Can you work these out from the model? Positions are in its coordinate system, mm. Round coordinates to 2 decimals unless told otherwise and drop trailing zeros. Loops run counter-clockwise (first coordinate to the right, second up) from the corner with the lowest first, then second, coordinate; pieces in that order, holes last. Notation, with made-up numbers: M -29.5,-12 L 2.5,-12 A8 cw 2.5,-5 Z; hole C 89,27 d9. An arc over 180 degrees is marked long. Answer as CSV lines item,"result".
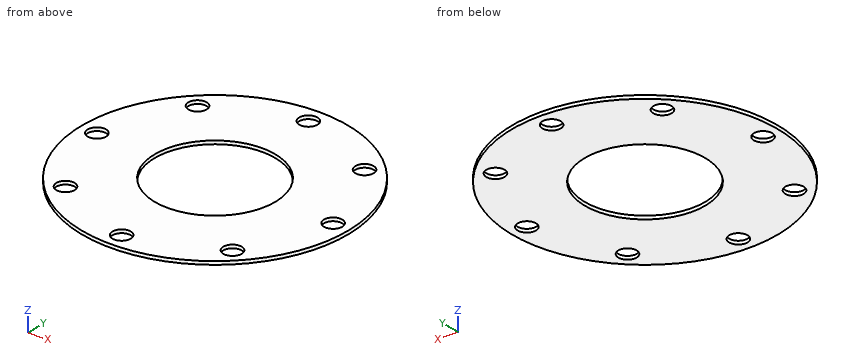
Autodesk Inventor part; units mm, degrees
ref_plane "YZ Plane" through (0, 0, 0) normal (1, 0, 0) x (0, 1, 0)
ref_plane "XZ Plane" through (0, 0, 0) normal (0, 1, 0) x (-1, 0, 0)
ref_plane "XY Plane" through (0, 0, 0) normal (0, 0, 1) x (1, 0, 0)
sketch "Sketch1" plane through (0, 0, 0) normal (0, 0, 1) x (1, 0, 0)
  circle A0 centre (0, 0) radius 72.5
  circle A1 centre (0, 0) radius 160
  dimension "d22" = 145
  dimension "d23" = 320
extrude "Plate1" add sketch "Sketch1" along normal blind 4
sketch "Sketch5" plane through (0, 0, 4) normal (0, 0, 1) x (1, 0, 0)
  circle A0 centre (0, 140) radius 11
  circle A1 centre (0, 0) radius 140 construction
  circle A2 centre (0, 0) radius 190 construction
  circle A3 centre (0, 190) radius 6.5
  dimension "d25" = 280
  dimension "d32" = 380
  dimension "d24" = 22
  dimension "d31" = 13
extrude "Cut1" cut sketch "Sketch5" against normal blind 4 contours A0
pattern_circular "Circular Pattern1" count 8 over 360 about axis through (0, 0, 0) along (0, 0, 1) of "Cut1"
equation "\"d26\" = Thickness"
equation "\"d2\" = Thickness"
equation "\"BendReliefWidth\" = Thickness"
equation "\"BendReliefDepth\" = 0.5 * Thickness"
equation "\"CornerReliefSize\" = 4 * Thickness"
equation "\"MinimumRemnant\" = 2 * Thickness"
equation "\"TransitionRadius\" = BendRadius"
equation "\"JacobiRadiusSize\" = BendRadius"
equation "\"GapSize\" = Thickness"
properties part number "TKS 3109 top DS main flange" material "Stainless Steel"
Item 1: If we section it at D-D on y = 60: Write out the boundary of the cut face in (x, z), then the cut area to 3 significant figures.
Output:
outline,"M -148.32,0 L -40.7,0 L -40.7,4 L -148.32,4 Z; M 40.7,0 L 148.32,0 L 148.32,4 L 40.7,4 Z"
area,"861 mm2"
Item 2: Will these pins go through, and if not, where does the flat tip stop? pin 1 (1.5 mm diameter, centred on x = -65.5, z = 0.5, fed in from +Y); pin 2 (1.5 mm diameter, centred on y = -79.5, z = 0.5, fed in from +X).
Output:
pin 1,"stops at y = 146.31"
pin 2,"stops at x = 139.28"
Item 3: If we section it at B-B on x = 140: Write out the boundary of the cut face in (y, z), then the cut area to 3 significant figures.
Output:
outline,"M -77.46,0 L -11,0 L -11,4 L -77.46,4 Z; M 11,0 L 77.46,0 L 77.46,4 L 11,4 Z"
area,"532 mm2"
Item 4: If I drill on line 1 along Y through (x, z) = (0, 1.9); line 2 along Y through (x, z) = (95.5, 1.25); line 3 along X through (y, z) = (91, 0.9), over which ranges is the centre line in solid material (lowest first)? Write a range as from..to.
Output:
line 1,"y = -160..-151, -129..-72.5, 72.5..129, 151..160"
line 2,"y = -128.37..-109.42, -88.56..88.56, 109.42..128.37"
line 3,"x = -131.6..-106.55, -91.44..91.44, 106.55..131.6"
Item 5: If we section it at A-A on y = 0: Write out the boundary of the cut face in (x, z).
Output:
outline,"M -160,0 L -151,0 L -151,4 L -160,4 Z; M -129,0 L -72.5,0 L -72.5,4 L -129,4 Z; M 72.5,0 L 129,0 L 129,4 L 72.5,4 Z; M 151,0 L 160,0 L 160,4 L 151,4 Z"
